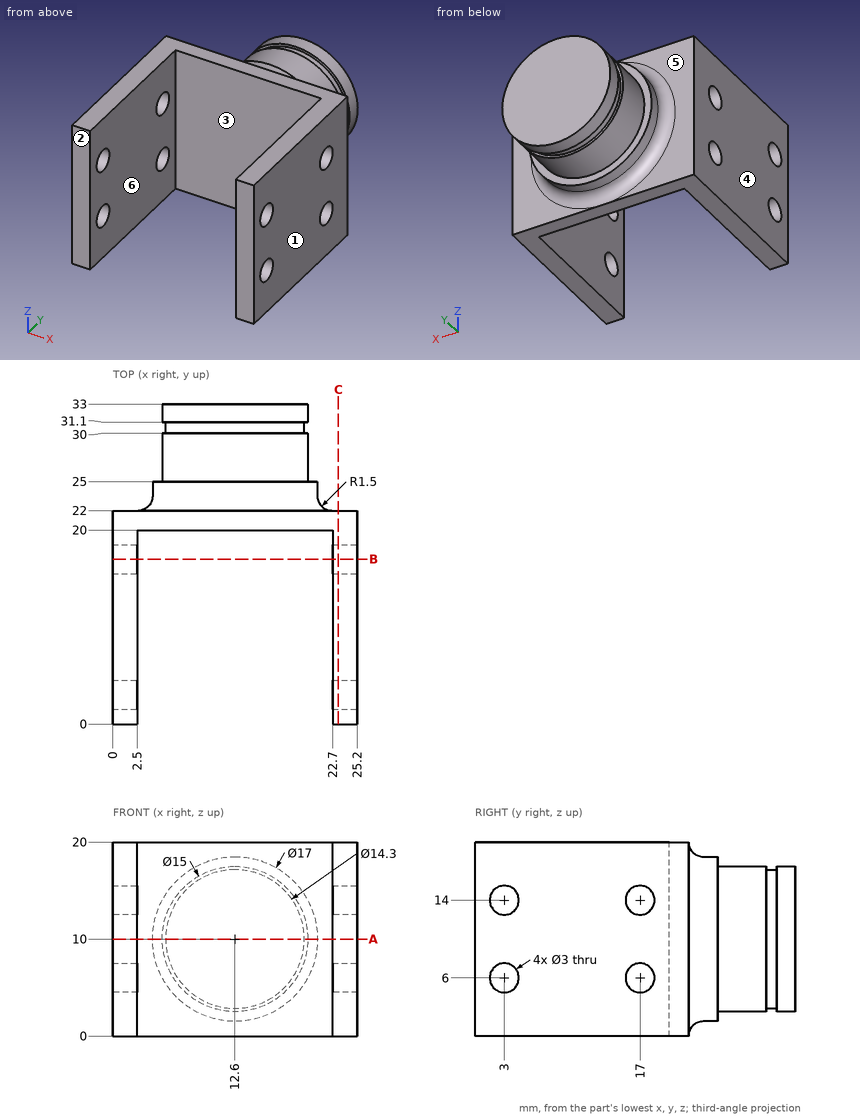
Print and shaded views of the part. All mm, measured from the part's lowest x, y and z. A direction names the side the tool comes from. Round coordinates to 2 decimals unless told otherwise and drop trailing zeros. Write each loop counter-clockwise with the first axis right and the second up, starting at its lowest first coordinate (ties: lowest second). Pieces come first, ordered by that corner, then holes. Notation, with made-up numbers: (5.25, 81) -> (54.25, 81) arc R34 ccw to (54.25, 117) -> close; hole circle Ø4 at (-16, -26). An arc over 180 degrees is marked (long way). Return JSON: item names as keys, results as strings. Group by question number.
Q1. Saw through at C-C on x = 23.25. Write the cut outline in (y, z), plus the area to 3 significant figures.
Q2. Probe L1, parallel to Y at x = 23.75, z = 6; L2, parallel to X at y = 5.5, z = 1; L3, parallel to Y at x = 2.75, z = 13. List the from-to ranges inside material, lowest first. Write a range as [from, to].
Q3. Saw through at A-A on z = 10. Write the cut outline in (x, y), plus the area to 3 significant figures.
Q4. Pin check, flat tips, straight feed: pin 1 (1 mm diameter, centred on x = 18, z = 17.5, fed in from +Y); pin 2 (2.5 mm diameter, centred on y = 3, z = 14, fed in from -X); pin 3 (12 mm diameter, centred on x = 11, z = 13, fed in from -Y). Stop position of each tip, or through.
Q5. Saw through at B-B on y = 17. Write the cut outline in (x, z).
Q6. Which spindle directions (+Z, -Z, +X, -X, +Y, -Y) get a long thin tool onto all of the face, cutting with end or side? Do the marked faces 4, 5 and 6. Say none if no direction does.
Q7. Mould opens along X. For the marked faces 1, 2 and 3 say: pulls with the +X half, pulls with the -X half, needs draft (parallel to the pull), parting line crosses it, or undercut.
Answer:
{
 "1": {"outline": "(0, 0) -> (22, 0) -> (22, 20) -> (0, 20) -> close; hole circle Ø3 at (3, 6); hole circle Ø3 at (3, 14); hole circle Ø3 at (17, 6); hole circle Ø3 at (17, 14)", "area": "412 mm2"},
 "2": {"L1": "[0, 1.5], [4.5, 15.5], [18.5, 22]", "L2": "[0, 2.5], [22.7, 25.2]", "L3": "[20, 22]"},
 "3": {"outline": "(0, 0) -> (2.5, 0) -> (2.5, 20) -> (22.7, 20) -> (22.7, 0) -> (25.2, 0) -> (25.2, 22) -> (22.6, 22) arc R1.5 cw to (21.1, 23.5) -> (21.1, 25) -> (20.1, 25) -> (20.1, 30) -> (19.75, 30) -> (19.75, 31.1) -> (20.1, 31.1) -> (20.1, 33) -> (5.1, 33) -> (5.1, 31.1) -> (5.45, 31.1) -> (5.45, 30) -> (5.1, 30) -> (5.1, 25) -> (4.1, 25) -> (4.1, 23.5) arc R1.5 cw to (2.6, 22) -> (0, 22) -> close", "area": "322 mm2"},
 "4": {"pin 1": "y = 22.68", "pin 2": "through", "pin 3": "y = 20"},
 "5": {"outline": "(0, 0) -> (2.5, 0) -> (2.5, 4.5) -> (0, 4.5) -> close; (0, 7.5) -> (2.5, 7.5) -> (2.5, 12.5) -> (0, 12.5) -> close; (0, 15.5) -> (2.5, 15.5) -> (2.5, 20) -> (0, 20) -> close; (22.7, 0) -> (25.2, 0) -> (25.2, 4.5) -> (22.7, 4.5) -> close; (22.7, 7.5) -> (25.2, 7.5) -> (25.2, 12.5) -> (22.7, 12.5) -> close; (22.7, 15.5) -> (25.2, 15.5) -> (25.2, 20) -> (22.7, 20) -> close"},
 "6": {"face 4": "+Z, -Z, -X, +Y, -Y", "face 5": "+Y", "face 6": "+Z, -Z, -Y"},
 "7": {"face 1": "pulls with the +X half", "face 2": "needs draft", "face 3": "undercut"}
}
